Design review of the part built by this model. Coordinates are the model's own, in mm. A direction names the side the tool comes from. Coordinates: 2 decimals unless noted, no trailing zeros. Loops run counter-clockwise (first coordinate to the right, second up) from the corner with the lowest first, then second, coordinate; pieces in that order, holes last. Notation, with made-up numbers: M 17.25,17.25 L 73.25,17.25 A26 ccw 73.25,32.25 Z; hole C 2,61.5 d4. An arc over 180 degrees is marked long. Answer as a JSON object with one key per item and string values. Group by question number.
1. Insertion check: pin 1 (6 mm diameter, centred on x = 15.5, z = 21.5, fed in from -Y); pin 2 (1.5 mm diameter, centred on x = 18.5, y = -1, fed in from -Z); pin 3 (3 mm diameter, centred on y = 6, z = 2, fed in from +X). Each pin has a flat end and moves straight along its axis. Give the tip position at first contact, or say it passes through.
2. Consider section C-C (x = 4). State the section outline as (y, z) points.
3. To check wall thickness, follow probe 1 along Y at (x, z) = (0, -1.85) (3 decimals); probe 2 along X at (y, z) = (-8.25, 30); probe 3 along Z at (x, y) = (2.5, 9). State the ranges of each line that lie inside material, in increasing order.
4. Draft analysis for pull direction Y (two halves, no side actions). For faces 3 (the flat face through (4, 0, -5.08)), 4 (the cylindrical face through (-0.69, -3.1, -2.5)), 5 (the cylindrical face through (20.284, -0.223, 37.585)), state which applies: +Y half, -Y half, draft (parallel to the pull), parting line (faces both ways), or undercut.
5. Machinability: for faces 1 (the flat face through (4, 0, 0)), 2 (the flat face through (22.86, 0, 21)), which of the approach directions +Z, -Z, +X, -X, +Y, -Y give a long, thin tool a straight path to every point of the face, cutting with its end or side? Answer none if there is none.
6. Consider section A-A (y = 0). State the section outline as (x, z) points (3 decimals), then the cut area to 3 significant figures.
7. Consider section B-B (z = 15.5). State the section outline as (x, y) points.
8. Consider section D-D (y = -4.25). State the section outline as (x, z) points, then the cut area to 3 significant figures.
Autodesk Inventor part; units mm, degrees
ref_plane "YZ Plane" through (0, 0, 0) normal (1, 0, 0) x (0, 1, 0)
ref_plane "XZ Plane" through (0, 0, 0) normal (0, 1, 0) x (-1, 0, 0)
ref_plane "XY Plane" through (0, 0, 0) normal (0, 0, 1) x (1, 0, 0)
sketch "Sketch1" plane through (0, 0, 0) normal (0, 0, 1) x (1, 0, 0)
  circle A0 centre (0, 0) radius 10.16
  line L0 (0, 10.16) -> (12.7, 10.16)
  line L1 (12.7, 10.16) -> (12.7, -10.16)
  line L2 (12.7, -10.16) -> (0, -10.16)
  line L3 (0, -10.16) -> (0, 10.16)
  circle A1 centre (0, 0) radius 3.175
  line L4 (12.7, 10.16) -> (27.7876, 10.16)
  line L5 (27.7876, 10.16) -> (27.7876, -10.16)
  line L6 (27.7876, -10.16) -> (12.7, -10.16)
  line L7 (12.7, -10.16) -> (12.7, 10.16)
  line L8 (27.7876, 10.16) -> (43.0276, 10.16)
  line L9 (43.0276, 10.16) -> (43.0276, -10.16)
  line L10 (43.0276, -10.16) -> (27.7876, -10.16)
  line L11 (27.7876, -10.16) -> (27.7876, 10.16)
  circle A2 centre (43.0276, 0) radius 10.16
  circle A3 centre (43.0276, 0) radius 3.175
  point P0 (0, -10.16)
  point P1 (12.7, -10.16)
  point P2 (43.0276, -10.16)
  dimension "d0" = 20.32
  dimension "d1" = 6.35
  dimension "d2" = 12.7
  dimension "d5" = 15.0876
  dimension "d6" = 15.24
extrude "Extrusion1" add sketch "Sketch1" against normal blind 5.08 contours A0 L3 A1 | A0 L0 L1 L2 | L3 A1 A0 | L4 L5 L6 L1 | L8 A2 L10 L5 | A2 L9 A3 | L9 A3 A2
sketch "Sketch2" plane through (0, 0, 0) normal (0, 0, 1) x (1, 0, 0)
  line L0 (12.7, -10.16) -> (12.7, 10.16)
  point P0 (0, 0)
bend part "Bend Part1" radius 5.08 angle 90 line through (12.7, -10.16, 0) along (0, 1, 0) centre toward (0, 0, 1) moving side (1, 0, 0) both sides no
sketch "Sketch3" plane through (22.86, 0, 27.428) normal (1, 0, 0) x (0, 0, -1)
  line L0 (32.508, -10.16) -> (32.508, 10.16)
  line L1 (17.4204, -10.16) -> (17.4204, 10.16)
  line L2 (0, 10.16) -> (22.348, 10.16)
  point P0 (27.428, 0)
  dimension "d10" = 15.0876
equation "\"d10\" = d5"
properties part number "ForearmActuatorBracketLeft"
Findings below:
{
 "1": {"pin 1": "stops at y = -10.16", "pin 2": "stops at z = -3.74", "pin 3": "stops at x = 22.74"},
 "2": {"outline": "M -10.16,-5.08 L 10.16,-5.08 L 10.16,0 L -10.16,0 Z"},
 "3": {"probe 1": "y = -10.16 to -3.175, 3.175 to 10.16", "probe 2": "x = 17.78 to 22.86", "probe 3": "z = -5.08 to 0"},
 "4": {"face 3": "draft", "face 4": "undercut", "face 5": "parting line"},
 "5": {"face 1": "+Z, -X, +Y, -Y", "face 2": "+Z, -Z, +X, +Y, -Y"},
 "6": {"outline": "M -10.16,-5.08 L -3.175,-5.08 L -3.175,0 L -10.16,0 Z; M 3.175,-5.08 L 12.7,-5.08 A10.16 ccw 22.86,5.08 L 22.86,24.253 L 17.78,24.253 L 17.78,5.08 A5.08 cw 12.7,0 L 3.175,0 Z; M 17.78,30.603 L 22.86,30.603 L 22.86,37.588 L 17.78,37.588 Z", "area": "278 mm^2"},
 "7": {"outline": "M 17.78,-10.16 L 22.86,-10.16 L 22.86,10.16 L 17.78,10.16 Z"},
 "8": {"outline": "M -9.23,-5.08 L 12.7,-5.08 A10.16 ccw 22.86,5.08 L 22.86,36.66 L 17.78,36.66 L 17.78,5.08 A5.08 cw 12.7,0 L -9.23,0 Z", "area": "333 mm^2"}
}
